Solid Edge part; units mm, degrees
sketch "Sketch1" plane through (0, 0, 0) normal (0, 0, 1) x (1, 0, 0)
  line L0 (2.75, -4) -> (2.75, 4)
  line L1 (2.75, 4) -> (-2.75, 4)
  line L2 (-2.75, 4) -> (-2.75, -4)
  line L3 (-2.75, -4) -> (2.75, -4)
extrude "Protrusion1" add sketch "Sketch1" along normal blind 11.2
hole "Hole_1" at (2.75, 0, 7.2) direction (-1, 0, 0) diameter 3 end up to next
Here's how the part is built. I have some questions about the finished solid (model axes, mm). Round coordinates to 2 decimals unless told otherwise and drop trailing zeros. Order: outer loops, then holes, each group sorted by start corner. A loop starts at its lowest first (then second) coordinate and runs counter-clockwise, first axis right, second up. Notation, with made-up numbers: (-24.5, 67) -> (6.5, 67) arc R16 ccw to (6.5, 90) -> close; hole circle Ø5 at (32.25, -8.75). An arc over 180 degrees is marked (long way). Use a Markdown table: item, result. Add a question column.
(1) I need wall thicknesses on line 1 along Z through (x, y) = (1.4, 0); line 2 along Y through (x, z) = (-1, 7.2); line 3 along Z through (x, y) = (-1.55, -0.5). Which ranges of each line are inside material? Lowest first, please.
(2) If we mould it in two halves opening along Z, with no side actions, what happens to faces 1 (the face through (0.04, 0.07, 8.7)), 2 (the face through (0, 0, 11.2)), 3 (the face through (0, 4, 6))? For each: released by +Z, released by -Z, zero draft, split by the parting line, or undercut.
(3) Suppose I cut it at B-B, the plane y = 0. Please give me the cut outline in (x, z).
(4) Suppose I cut it at A-A, the plane z = 7.2. Please give me the cut outline in (x, y).
(5) Suppose I cut it at C-C, the plane x = -1.65. Please give me the cut outline in (y, z).
Verdict:
| question | item | result |
|---|---|---|
| 1 | line 1 | 0 to 5.7, 8.7 to 11.2 |
| 1 | line 2 | -4 to -1.5, 1.5 to 4 |
| 1 | line 3 | 0 to 5.79, 8.61 to 11.2 |
| 2 | face 1 | undercut |
| 2 | face 2 | released by +Z |
| 2 | face 3 | zero draft |
| 3 | outline | (-2.75, 0) -> (2.75, 0) -> (2.75, 5.7) -> (-2.75, 5.7) -> close; (-2.75, 8.7) -> (2.75, 8.7) -> (2.75, 11.2) -> (-2.75, 11.2) -> close |
| 4 | outline | (-2.75, -4) -> (2.75, -4) -> (2.75, -1.5) -> (-2.75, -1.5) -> close; (-2.75, 1.5) -> (2.75, 1.5) -> (2.75, 4) -> (-2.75, 4) -> close |
| 5 | outline | (-4, 0) -> (4, 0) -> (4, 11.2) -> (-4, 11.2) -> close; hole circle Ø3 at (0, 7.2) |
